Here's the drawing with two shaded views (mm, measured from the low corner). I have some questions. A direction names the side the tool comes from. Coordinates: 2 decimals unless noted, no trailing zeros. Write each loop counter-clockwise with the first axis right and the second up, starting at its lowest first coordinate (ties: lowest second). Pieces come first, ordered by that corner, then holes.
Item 1: We'd pull the mould along Z, two halves only. Please class the marked faces 3, 4, 5 and 6: +Z half, -Z half, draft (parallel to the pull), parting line (faces both ways), or undercut.
Item 2: If I drill on line 1 (Y direction, x = 7, z = 42); line 2 (X direction, y = 52.5, z = 25); line 3 (Z direction, x = 41, y = 30.5) (1 decimal), over which ranges is the centre line in solid material (lowest first)?
Item 3: If we section it at B-B (z = 24): Please give me the cut outline in (x, y) (1 decimal).
Item 4: If we section it at A-A (y = 19): Please give me the cut outline in (x, z), then the cut area to 3 significant figures.
Item 5: If we section it at C-C (x = 24.5): Please give me the cut outline in (y, z), then the cut area to 3 significant figures.
Item 6: For the marked faces 1 and 2, which set-ups out of +Z, -Z, +X, -X, +Y, -Y let a thin tool reach every point of the face, with its end or its side?
Item 7: If we section it at D-D (y = 27.5): Please give me the cut outline in (x, z).
Item 8: I'm going to push flat-ended pins straight in: pin 1 Ø5 at (x, z) = (36.5, 13) entering from +Y; pin 2 Ø6.5 at (y, z) = (55.5, 23.5) entering from +X; pin 3 Ø10 at (x, y) = (30.5, 59) entering from -Z. Where does each tip first touch, or does it pass through?
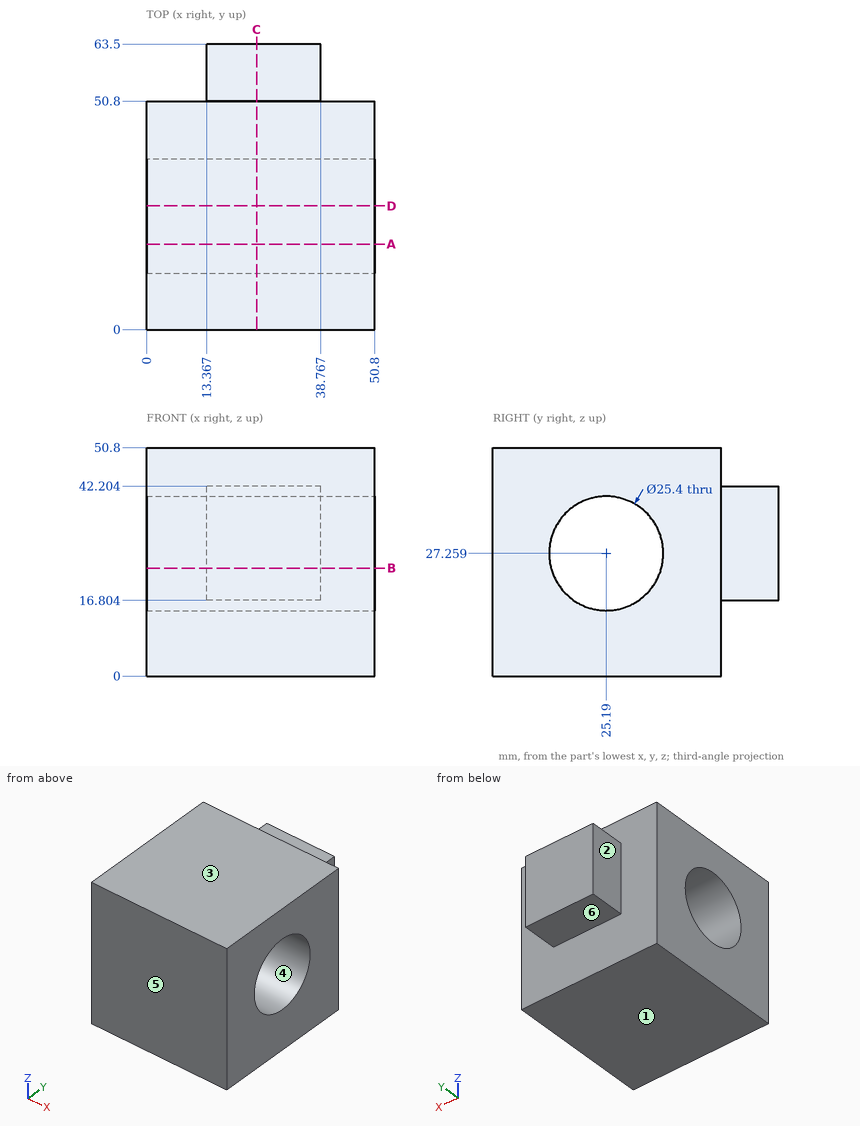
Answer list:
1. face 3: +Z half
1. face 4: undercut
1. face 5: draft
1. face 6: -Z half
2. line 1: y = 0 to 50.8
2. line 2: x = 13.37 to 38.77
2. line 3: z = 0 to 15.7, 38.8 to 50.8
3. outline: (0, 0) - (50.8, 0) - (50.8, 12.9) - (0, 12.9) - close; (0, 37.5) - (50.8, 37.5) - (50.8, 50.8) - (38.8, 50.8) - (38.8, 63.5) - (13.4, 63.5) - (13.4, 50.8) - (0, 50.8) - close
4. outline: (0, 0) - (50.8, 0) - (50.8, 16.17) - (0, 16.17) - close; (0, 38.35) - (50.8, 38.35) - (50.8, 50.8) - (0, 50.8) - close
4. area: 1,450 mm2
5. outline: (0, 0) - (50.8, 0) - (50.8, 16.8) - (63.5, 16.8) - (63.5, 42.2) - (50.8, 42.2) - (50.8, 50.8) - (0, 50.8) - close; hole circle Ø25.4 at (25.19, 27.26)
5. area: 2,400 mm2
6. face 1: -Z, +X, -X, +Y, -Y
6. face 2: +Z, -Z, -X, +Y
7. outline: (0, 0) - (50.8, 0) - (50.8, 14.77) - (0, 14.77) - close; (0, 39.75) - (50.8, 39.75) - (50.8, 50.8) - (0, 50.8) - close
8. pin 1: stops at y = 50.8
8. pin 2: stops at x = 38.77
8. pin 3: stops at z = 16.8
